```python
from build123d import *

# Parameters (mm, degrees)
ESQUISSE1_W                        = 100
ESQUISSE1_H                        = 35
BOSS_EXTRU_1_DEPTH                 = 3
ESQUISSE2_R                        = 1.5
ENL_V_MAT_EXTRU_1_DEPTH            = 3
CONG_1_R                           = 1
R_P_TITION_CIRCULAIRE4_COUNT       = 2
R_P_TITION_CIRCULAIRE4_ANGLE       = 90
R_P_TITION_CIRCULAIRE4_2_COUNT     = 2
R_P_TITION_CIRCULAIRE4_2_ANGLE     = 90
CONG_1_OF_R_P_TITION_CIRCULAIRE4_R = 1
ESQUISSE4_R                        = 1.5
ENL_V_MAT_EXTRU_2_DEPTH            = 10
CONG_2_R                           = 1


with BuildPart() as part:
    # Esquisse1 → Boss.-Extru.1 (new body)
    with BuildSketch(Plane.XY):
        with Locations((50, 17.5)):
            Rectangle(ESQUISSE1_W, ESQUISSE1_H)
    boss_extru_1 = extrude(amount=BOSS_EXTRU_1_DEPTH)

    # Esquisse2 → Enlèv. mat.-Extru.1 (cut)
    with BuildSketch(Plane.XY.offset(3)):
        with Locations((95, 32.5)):
            Circle(ESQUISSE2_R)
        with Locations((85, 32.5)):
            Circle(ESQUISSE2_R)
        with Locations((75, 32.5)):
            Circle(ESQUISSE2_R)
        with Locations((65, 32.5)):
            Circle(ESQUISSE2_R)
        with Locations((55, 32.5)):
            Circle(ESQUISSE2_R)
        with Locations((45, 32.5)):
            Circle(ESQUISSE2_R)
        with Locations((85, 22.5)):
            Circle(ESQUISSE2_R)
        with Locations((75, 22.5)):
            Circle(ESQUISSE2_R)
        with Locations((65, 22.5)):
            Circle(ESQUISSE2_R)
        with Locations((55, 22.5)):
            Circle(ESQUISSE2_R)
        with Locations((45, 22.5)):
            Circle(ESQUISSE2_R)
        with Locations((85, 12.5)):
            Circle(ESQUISSE2_R)
        with Locations((75, 12.5)):
            Circle(ESQUISSE2_R)
        with Locations((65, 12.5)):
            Circle(ESQUISSE2_R)
        with Locations((55, 12.5)):
            Circle(ESQUISSE2_R)
        with Locations((45, 12.5)):
            Circle(ESQUISSE2_R)
        with Locations((85, 2.5)):
            Circle(ESQUISSE2_R)
        with Locations((75, 2.5)):
            Circle(ESQUISSE2_R)
        with Locations((65, 2.5)):
            Circle(ESQUISSE2_R)
        with Locations((55, 2.5)):
            Circle(ESQUISSE2_R)
        with Locations((45, 2.5)):
            Circle(ESQUISSE2_R)
        with Locations((95, 22.5)):
            Circle(ESQUISSE2_R)
        with Locations((95, 12.5)):
            Circle(ESQUISSE2_R)
        with Locations((95, 2.5)):
            Circle(ESQUISSE2_R)
    enl_v_mat_extru_1 = extrude(amount=-ENL_V_MAT_EXTRU_1_DEPTH, mode=Mode.SUBTRACT)

    # Congé1
    cong_1_edges = [part.edges().sort_by_distance(p)[0] for p in [
        (0, 35, 1.5),
        (100, 35, 1.5),
        (100, 0, 1.5),
        (0, 0, 1.5),
    ]]
    fillet(cong_1_edges, radius=CONG_1_R)


with BuildPart() as r_p_tition_circulaire4_1:
    # Répétition circulaire4: Boss.-Extru.1 ×2 about axis
    r_p_tition_circulaire4_axis = Axis((17.5, 17.5, 0), (0, 0, 1))
    for i in range(1, R_P_TITION_CIRCULAIRE4_COUNT):
        add(boss_extru_1.rotate(r_p_tition_circulaire4_axis, i * R_P_TITION_CIRCULAIRE4_ANGLE / (R_P_TITION_CIRCULAIRE4_COUNT - 1)))

    # R_p_tition circulaire4 2: Enlèv. mat.-Extru.1 ×2 about axis
    r_p_tition_circulaire4_2_axis = Axis((17.5, 17.5, 0), (0, 0, 1))
    for i in range(1, R_P_TITION_CIRCULAIRE4_2_COUNT):
        add(enl_v_mat_extru_1.rotate(r_p_tition_circulaire4_2_axis, i * R_P_TITION_CIRCULAIRE4_2_ANGLE / (R_P_TITION_CIRCULAIRE4_2_COUNT - 1)), mode=Mode.SUBTRACT)

    # Congé1 of Répétition circulaire4
    cong_1_of_r_p_tition_circulaire4_edges = [r_p_tition_circulaire4_1.edges().sort_by_distance(p)[0] for p in [
        (0, 0, 1.5),
        (0, 100, 1.5),
        (35, 100, 1.5),
        (35, 0, 1.5),
    ]]
    fillet(cong_1_of_r_p_tition_circulaire4_edges, radius=CONG_1_OF_R_P_TITION_CIRCULAIRE4_R)


with BuildPart() as part_1:
    add(part.part)

    # Répétition circulaire4 united with what: union Répétition circulaire4_1
    add(r_p_tition_circulaire4_1.part)

    # Esquisse4 → Enlèv. mat.-Extru.2 (cut)
    with BuildSketch(Plane.XY.offset(3)):
        with Locations((2.5, 2.5)):
            Circle(ESQUISSE4_R)
        with Locations((12.5, 2.5)):
            Circle(ESQUISSE4_R)
        with Locations((22.5, 2.5)):
            Circle(ESQUISSE4_R)
        with Locations((32.5, 2.5)):
            Circle(ESQUISSE4_R)
        with Locations((12.5, 12.5)):
            Circle(ESQUISSE4_R)
        with Locations((22.5, 12.5)):
            Circle(ESQUISSE4_R)
        with Locations((32.5, 12.5)):
            Circle(ESQUISSE4_R)
        with Locations((12.5, 22.5)):
            Circle(ESQUISSE4_R)
        with Locations((22.5, 22.5)):
            Circle(ESQUISSE4_R)
        with Locations((32.5, 22.5)):
            Circle(ESQUISSE4_R)
        with Locations((12.5, 32.5)):
            Circle(ESQUISSE4_R)
        with Locations((22.5, 32.5)):
            Circle(ESQUISSE4_R)
        with Locations((32.5, 32.5)):
            Circle(ESQUISSE4_R)
        with Locations((2.5, 12.5)):
            Circle(ESQUISSE4_R)
        with Locations((2.5, 22.5)):
            Circle(ESQUISSE4_R)
        with Locations((2.5, 32.5)):
            Circle(ESQUISSE4_R)
    extrude(amount=-ENL_V_MAT_EXTRU_2_DEPTH, mode=Mode.SUBTRACT)

    # Congé2
    cong_2_edges = [part_1.edges().sort_by_distance(p)[0] for p in [
        (67, 35, 0),
        (100, 17.5, 0),
        (99.707106781, 34.707106781, 0),
        (99.707106781, 0.292893219, 0),
        (67, 35, 3),
        (100, 17.5, 3),
        (99.707106781, 34.707106781, 3),
        (99.707106781, 0.292893219, 3),
        (35, 35, 1.5),
        (35, 67, 0),
        (35, 67, 3),
        (50, 0, 0),
        (50, 0, 3),
        (0, 50, 0),
        (17.5, 100, 0),
        (0.292893219, 99.707106781, 0),
        (34.707106781, 99.707106781, 0),
        (0.292893219, 0.292893219, 0),
        (0, 50, 3),
        (17.5, 100, 3),
        (0.292893219, 99.707106781, 3),
        (34.707106781, 99.707106781, 3),
        (0.292893219, 0.292893219, 3),
    ]]
    fillet(cong_2_edges, radius=CONG_2_R - 0.0001)  # a hair under: the kernel refuses the full size


solid = part_1.part
```
The model under review builds one solid part; all positions refer to its coordinate system, in mm. Round coordinates to 2 decimals unless told otherwise and drop trailing zeros. Order: outer loops, then holes, each group sorted by start corner. A loop starts at its lowest first (then second) coordinate and runs counter-clockwise, first axis right, second up. Notation, with made-up numbers: M 51.25,50 L 72.25,50 A19 cw 72.25,70 Z; hole C 5,10 d8. An arc over 180 degrees is marked long. Use a Markdown table: item, result.
1) Insertion check: pin 1 (2.5 mm diameter, centred on x = 95, y = 12.5, fed in from -Z); pin 2 (1.5 mm diameter, centred on y = 36, z = 1.5, fed in from +X). Each pin has a flat end and moves straight along its axis. Give the tip position at first contact, or say it passes through.
Report:
| item | result |
|---|---|
| pin 1 | through |
| pin 2 | x = 35.34 |
2) Draft analysis for pull direction Y (two halves, no side actions). For faces 1 (the face through (95.69, 31.17, 1.52)), 2 (the face through (38, 29, 0)), state which applies: released by +Y, released by -Y, zero draft, split by the parting line, or undercut.
Report:
| item | result |
|---|---|
| face 1 | undercut |
| face 2 | zero draft |
3) Consider section A-A (y = 55). Give the number of separate pieces and of enclosed holes in the cut face, then the cut area to 3 significant figures.
Report:
| item | result |
|---|---|
| separate pieces | 5 |
| enclosed holes | 0 |
| area | 68.1 mm^2 |
4) Consider section C-C (x = 51.5). Write out the cut boundary in (y, z).
Report:
| item | result |
|---|---|
| outline | M 0,1 A1 ccw 1,0 L 34,0 A1 ccw 35,1 L 35,2 A1 ccw 34,3 L 1,3 A1 ccw 0,2 Z |
5) Wall thickness on line 1 along Y through (x, z) = (45, 0.85); line 2 along X through (y, z) = (45, 1.2); line 3 along Y through (x, z) = (54.5, 2.2): over which ranges is each line inside the solid? List them lowest first. Write a range as [from, to].
Report:
| item | result |
|---|---|
| line 1 | [0.01, 1], [4, 11], [14, 21], [24, 31], [34, 34.99] |
| line 2 | [0, 1], [4, 11], [14, 21], [24, 31], [34, 35] |
| line 3 | [0.02, 1.09], [3.91, 11.09], [13.91, 21.09], [23.91, 31.09], [33.91, 34.98] |
